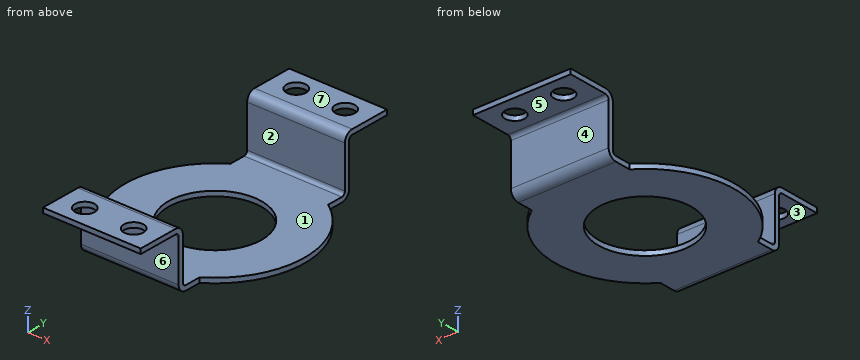
```python
from build123d import *

# Parameters (mm, degrees)
SKETCH_1_R                       = 9.5
SM_BASE_FLANGE_1_DEPTH           = 1
SM_EDGE_FLANGE_1_STRIP_W         = 5.4732
SM_EDGE_FLANGE_1_STRIP_H         = 1
SM_EDGE_FLANGE_1_STRIP_CUT_DEPTH = 20
SM_EDGE_FLANGE_1_DEPTH           = 20
SM_EDGE_FLANGE_2_STRIP_W         = 5.4732
SM_EDGE_FLANGE_2_STRIP_H         = 1
SM_EDGE_FLANGE_2_STRIP_CUT_DEPTH = 20
SM_EDGE_FLANGE_2_DEPTH           = 20
SM_EDGE_FLANGE_3_STRIP_W         = 5.4732
SM_EDGE_FLANGE_3_STRIP_H         = 1
SM_EDGE_FLANGE_3_STRIP_CUT_DEPTH = 20
SM_EDGE_FLANGE_3_DEPTH           = 20
SM_EDGE_FLANGE_4_STRIP_W         = 5.4732
SM_EDGE_FLANGE_4_STRIP_H         = 1
SM_EDGE_FLANGE_4_STRIP_CUT_DEPTH = 20
SM_EDGE_FLANGE_4_DEPTH           = 20
CUT_EXTRUDE_2_DEPTH              = 37.505136625
CUT_EXTRUDE_2_DEPTH_BACK         = 37.505136625
SKETCH_19_R                      = 2


# Sheet-metal steps are written as plain solids
with BuildPart() as part:
    # Sketch 1 → Базовая кромка1 (new body)
    with BuildSketch(Plane.XY):
        with BuildLine():
            Line((-10, 15.266384641), (-10, 20.25))
            Line((-10, 20.25), (10, 20.25))
            Line((10, 20.25), (10, 15.266384641))
            ThreePointArc((10, 15.266384641), (18.25, 0), (10, -15.266384641))
            Line((10, -15.266384641), (10, -20.25))
            Line((10, -20.25), (-10, -20.25))
            Line((-10, -20.25), (-10, -15.266384641))
            ThreePointArc((-10, -15.266384641), (-18.25, 0), (-10, 15.266384641))
        make_face()
        Circle(SKETCH_1_R, mode=Mode.SUBTRACT)
    extrude(amount=-SM_BASE_FLANGE_1_DEPTH)

    # Ребро-кромка1 strip (across the edge) → Ребро-кромка1 strip cut (cut)
    with BuildSketch(Plane(origin=(10, 20.25, 0), x_dir=(0, -1, 0), z_dir=(-1, 0, 0))):
        with Locations((-1, -0.5)):
            Rectangle(SM_EDGE_FLANGE_1_STRIP_W, SM_EDGE_FLANGE_1_STRIP_H)
    extrude(amount=SM_EDGE_FLANGE_1_STRIP_CUT_DEPTH, mode=Mode.SUBTRACT)

    # Ребро-кромка1 section (across the edge) → Ребро-кромка1 (add)
    with BuildSketch(Plane(origin=(10, 20.25, 0), x_dir=(0, -1, 0), z_dir=(-1, 0, 0))):
        with BuildLine():
            Line((0, 0.7366), (0, 11))
            Line((0, 11), (1, 11))
            Line((1, 11), (1, 0.7366))
            ThreePointArc((1, 0.7366), (1.215745145, 0.215745145), (1.7366, 0))
            Line((1.7366, 0), (1.7366, -1))
            ThreePointArc((1.7366, -1), (0.508638364, -0.491361636), (0, 0.7366))
        make_face()
    extrude(amount=SM_EDGE_FLANGE_1_DEPTH)

    # Ребро-кромка2 strip (across the edge) → Ребро-кромка2 strip cut (cut)
    with BuildSketch(Plane(origin=(-10, -20.25, 0), x_dir=(0, 1, 0), z_dir=(1, 0, 0))):
        with Locations((-1, -0.5)):
            Rectangle(SM_EDGE_FLANGE_2_STRIP_W, SM_EDGE_FLANGE_2_STRIP_H)
    extrude(amount=SM_EDGE_FLANGE_2_STRIP_CUT_DEPTH, mode=Mode.SUBTRACT)

    # Ребро-кромка2 section (across the edge) → Ребро-кромка2 (add)
    with BuildSketch(Plane(origin=(-10, -20.25, 0), x_dir=(0, 1, 0), z_dir=(1, 0, 0))):
        with BuildLine():
            Line((0, 0.7366), (0, 11))
            Line((0, 11), (1, 11))
            Line((1, 11), (1, 0.7366))
            ThreePointArc((1, 0.7366), (1.215745145, 0.215745145), (1.7366, 0))
            Line((1.7366, 0), (1.7366, -1))
            ThreePointArc((1.7366, -1), (0.508638364, -0.491361636), (0, 0.7366))
        make_face()
    extrude(amount=SM_EDGE_FLANGE_2_DEPTH)

    # Ребро-кромка3 strip (across the edge) → Ребро-кромка3 strip cut (cut)
    with BuildSketch(Plane(origin=(-10, 20.25, 11), x_dir=(0, 0, -1), z_dir=(1, 0, 0))):
        with Locations((-1, -0.5)):
            Rectangle(SM_EDGE_FLANGE_3_STRIP_W, SM_EDGE_FLANGE_3_STRIP_H)
    extrude(amount=SM_EDGE_FLANGE_3_STRIP_CUT_DEPTH, mode=Mode.SUBTRACT)

    # Ребро-кромка3 section (across the edge) → Ребро-кромка3 (add)
    with BuildSketch(Plane(origin=(-10, 20.25, 11), x_dir=(0, 0, -1), z_dir=(1, 0, 0))):
        with BuildLine():
            Line((0, 0.7366), (0, 9))
            Line((0, 9), (1, 9))
            Line((1, 9), (1, 0.7366))
            ThreePointArc((1, 0.7366), (1.215745145, 0.215745145), (1.7366, 0))
            Line((1.7366, 0), (1.7366, -1))
            ThreePointArc((1.7366, -1), (0.508638364, -0.491361636), (0, 0.7366))
        make_face()
    extrude(amount=SM_EDGE_FLANGE_3_DEPTH)

    # Ребро-кромка4 strip (across the edge) → Ребро-кромка4 strip cut (cut)
    with BuildSketch(Plane(origin=(10, -20.25, 11), x_dir=(0, 0, -1), z_dir=(-1, 0, 0))):
        with Locations((-1, -0.5)):
            Rectangle(SM_EDGE_FLANGE_4_STRIP_W, SM_EDGE_FLANGE_4_STRIP_H)
    extrude(amount=SM_EDGE_FLANGE_4_STRIP_CUT_DEPTH, mode=Mode.SUBTRACT)

    # Ребро-кромка4 section (across the edge) → Ребро-кромка4 (add)
    with BuildSketch(Plane(origin=(10, -20.25, 11), x_dir=(0, 0, -1), z_dir=(-1, 0, 0))):
        with BuildLine():
            Line((0, 0.7366), (0, 9))
            Line((0, 9), (1, 9))
            Line((1, 9), (1, 0.7366))
            ThreePointArc((1, 0.7366), (1.215745145, 0.215745145), (1.7366, 0))
            Line((1.7366, 0), (1.7366, -1))
            ThreePointArc((1.7366, -1), (0.508638364, -0.491361636), (0, 0.7366))
        make_face()
    extrude(amount=SM_EDGE_FLANGE_4_DEPTH)

    # Эскиз19 → Вырез-Вытянуть2 (cut, two sides: drawn at the far end of the back side and taken through both)
    with BuildSketch(Plane.XY.offset(11).offset(-CUT_EXTRUDE_2_DEPTH_BACK)):
        with Locations(Location((-5, 25.1183, 0), (0, 0, 180))):
            Circle(SKETCH_19_R)
        with Locations(Location((5, 25.1183, 0), (0, 0, 180))):
            Circle(SKETCH_19_R)
        with Locations(Location((5, -25.1183, 0), (0, 0, 180))):
            Circle(SKETCH_19_R)
        with Locations(Location((-5, -25.1183, 0), (0, 0, 180))):
            Circle(SKETCH_19_R)
    extrude(amount=CUT_EXTRUDE_2_DEPTH + CUT_EXTRUDE_2_DEPTH_BACK, mode=Mode.SUBTRACT)


solid = part.part
```
CAD build for the part. Positions are in the model's coordinates, mm. Face numbers are marked on the shaded views. A direction names the side the tool comes from. Coordinates: 2 decimals unless noted, no trailing zeros. Order: outer loops, then holes, each group sorted by start corner. A loop starts at its lowest first (then second) coordinate and runs counter-clockwise, first axis right, second up. Notation, with made-up numbers: (14, -30) - (52, -30) arc R7 ccw to (52, -17) - close; hole circle Ø5 at (-4, 77). An arc over 180 degrees is marked (long way). Answer in a Markdown table with one row per item.
1. Slice it at A-A, the plane z = 8.5. List the corners of the cut face in (x, y), then the cut area to 3 significant figures.
Answer:
| item | result |
|---|---|
| outline | (-10, -20.25) - (10, -20.25) - (10, -19.25) - (-10, -19.25) - close; (-10, 19.25) - (10, 19.25) - (10, 20.25) - (-10, 20.25) - close |
| area | 40.0 mm² |
2. 3-axis set-ups, long thin cutter, end or side, ignore diameter. For the marked faces 5, 6 and 7: which of +Z, -Z, +X, -X, +Y, -Y reach the whole face in a straight line?
Answer:
| item | result |
|---|---|
| face 5 | -Z, +X, -X, +Y |
| face 6 | -Z, +X, -X, -Y |
| face 7 | +Z, +X, -X, +Y, -Y |
3. Drill centre lines: L1, parallel to Y at x = 3.5, z = 0.75; L2, parallel to Y at x = 5, z = 10.35; L3, parallel to Y at x = 5, z = 10.6. Where is each one in solid material? Low to high. Write a range as from..to.
Answer:
| item | result |
|---|---|
| L1 | -20.25..-19.25, 19.25..20.25 |
| L2 | -29.25..-27.12, -23.12..-19.63, 19.63..23.12, 27.12..29.25 |
| L3 | -29.25..-27.12, -23.12..-19.88, 19.88..23.12, 27.12..29.25 |
4. Slice it at B-B, the plane y = 0. List the corners of the cut face in (x, z).
Answer:
| item | result |
|---|---|
| outline | (-18.25, -1) - (-9.5, -1) - (-9.5, 0) - (-18.25, 0) - close; (9.5, -1) - (18.25, -1) - (18.25, 0) - (9.5, 0) - close |
5. Slice it at C-C, the plane x = 0. List the corners of the cut face in (y, z), then the cut area to 3 significant figures.
Answer:
| item | result |
|---|---|
| outline | (-29.25, 10) - (-20.99, 10) arc R0.74 cw to (-20.25, 9.26) - (-20.25, 0.74) arc R1.74 ccw to (-18.51, -1) - (-9.5, -1) - (-9.5, 0) - (-18.51, 0) arc R0.74 cw to (-19.25, 0.74) - (-19.25, 9.26) arc R1.74 ccw to (-20.99, 11) - (-29.25, 11) - close; (9.5, -1) - (18.51, -1) arc R1.74 ccw to (20.25, 0.74) - (20.25, 9.26) arc R0.74 cw to (20.99, 10) - (29.25, 10) - (29.25, 11) - (20.99, 11) arc R1.74 ccw to (19.25, 9.26) - (19.25, 0.74) arc R0.74 cw to (18.51, 0) - (9.5, 0) - close |
| area | 59.4 mm² |
6. Pull direction Y, two halves, no side cores. Call the marked faces 1, 2, 3 and 4: +Y half, -Y half, draft (parallel to the pull), parting line (faces both ways), or undercut.
Answer:
| item | result |
|---|---|
| face 1 | undercut |
| face 2 | undercut |
| face 3 | draft |
| face 4 | +Y half |
7. Slice it at D-D, the plane x = 5. Give the number of separate pieces and of enclosed holes in the cut face, then the cut area to 3 significant figures.
Answer:
| item | result |
|---|---|
| separate pieces | 4 |
| enclosed holes | 0 |
| area | 54.2 mm² |
8. Flat gauge pins, fed straight in: P1, Ø7, axis at x = -3, z = 4, coming from the -Y side; P2, Ø1, axis at x = 9, z = 1.5, coming from the +Y side; P3, Ø5, axis at y = -18, z = 1.5, coming from the +X side; P4, Ø6, axis at x = -2.5, y = -2.5, coming from the -Z side. Where does each tip first touch, or does it go through?
Answer:
| item | result |
|---|---|
| P1 | y = -20.25 |
| P2 | y = 20.25 |
| P3 | x = 10 |
| P4 | through |
